Part print with two shaded views. Sizes in mm from the minimum x, y, z corner. A direction names the side the tool comes from. Coordinates: 2 decimals unless noted, no trailing zeros. Order: outer loops, then holes, each group sorted by start corner. A loop starts at its lowest first (then second) coordinate and runs counter-clockwise, first axis right, second up. Notation, with made-up numbers: (64.5, -16.5) - (84.5, -16.5) arc R28 ccw to (84.5, 15.5) - close; hole circle Ø11 at (0.25, 3.5). An arc over 180 degrees is marked (long way). Write each question's results on one line, items separated by ' | '. Start each with the question number.
Q1. Band-saw the part on C-C, the plane z = 16.5. Write the cut outline in (x, y).
Q2. Band-saw the part on D-D, the plane y = 7. Write the cut outline in (x, z), then the cut area to 3 significant figures.
Q3. Band-saw the part on A-A, the plane y = 14. Write the cut outline in (x, z).
Q4. Pull direction Z, two halves, no side cores. Call the marked faces 1, 2 and 3: released by +Z, released by -Z, zero draft, split by the parting line, or undercut.
Q5. Which spindle directions (+Z, -Z, +X, -X, +Y, -Y) get a long thin tool onto all of the face, cutting with end or side? Do the marked faces 4 and 5. Say none if no direction does.
Q6. Pin check, flat tips, straight feed: P1, Ø1, axis at y = 38, z = 22.5, coming from the +X side (1 decimal); P2, Ø3, axis at y = 12, z = 51.5, coming from the +X side; P3, Ø1.5, axis at x = 101.5, y = 5, coming from the +Z side. Stop position of each tip, or through.
Q7. Wall check: probe 1 along Z at (x, y) = (69.5, 19); probe 2 along Z at (x, y) = (31.5, 30.5) (1 decimal); probe 3 along X at (y, z) = (21, 50) (1 decimal). Give the ranges that are in metal, low to high.
Q8. Band-saw the part on B-B, the plane x = 117. Write the cut outline in (y, z), then the cut area to 3 significant figures.
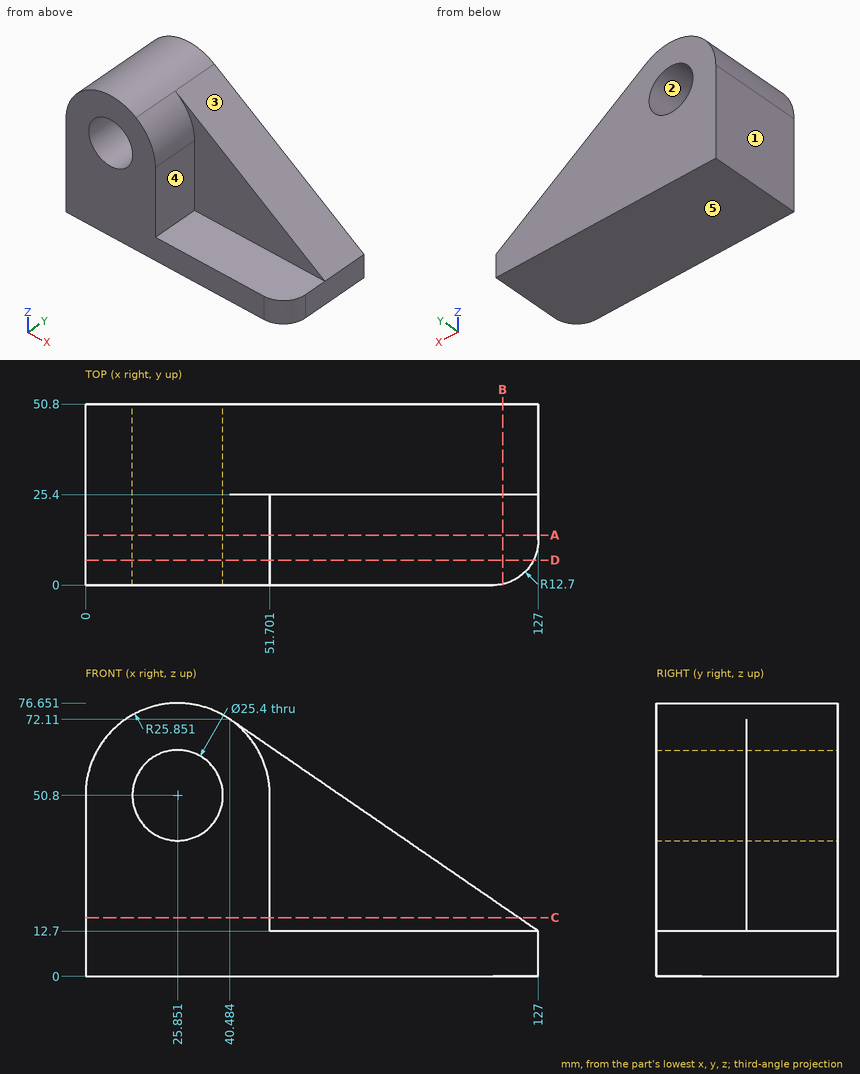
Results below:
1) outline: (0, 0) - (51.7, 0) - (51.7, 25.4) - (121.47, 25.4) - (121.47, 50.8) - (0, 50.8) - close
2) outline: (0, 0) - (125.65, 0) - (125.65, 12.7) - (51.7, 12.7) - (51.7, 50.8) arc R25.85 ccw to (40.48, 72.11) arc R25.85 ccw to (0, 50.8) - close; hole circle Ø25.4 at (25.85, 50.8) | area: 4,110 mm²
3) outline: (0, 0) - (127, 0) - (127, 12.7) - (51.7, 12.7) - (51.7, 50.8) arc R25.85 ccw to (40.48, 72.11) arc R25.85 ccw to (0, 50.8) - close; hole circle Ø25.4 at (25.85, 50.8)
4) face 1: zero draft | face 2: undercut | face 3: released by +Z
5) face 4: +Z, +X, -Y | face 5: -Z, +X, -X, +Y, -Y
6) P1: stops at x = 113.5 | P2: stops at x = 51.7 | P3: stops at z = 12.7
7) probe 1: z = 0 to 12.7 | probe 2: z = 0 to 39.4, 62.2 to 76 | probe 3: x = 0 to 13.2, 38.5 to 51.7
8) outline: (0.29, 0) - (50.8, 0) - (50.8, 19.57) - (25.4, 19.57) - (25.4, 12.7) - (0.29, 12.7) - close | area: 816 mm²
